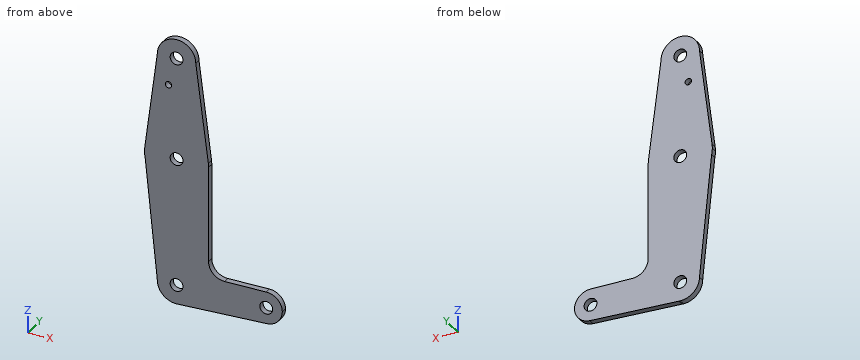
```python
from build123d import *

# Parameters (mm, degrees)
F0_R     = 3.175
F0_R_2   = 1.5875
F1_DEPTH = 3.048


with BuildPart() as f1:
    # F0 (on Front) → F1 (new body)
    with BuildSketch(Plane.XZ):
        with BuildLine():
            ThreePointArc((15.747457, 2.008289), (0, 15.875), (-15.747457, 2.008289))
            ThreePointArc((-15.747457, 2.008289), (-15.843082, 1.006168), (-15.875, 0))
            Line((-15.875, 0), (-15.560644, -3.143564))
            ThreePointArc((-15.560644, -3.143564), (1.579622, -15.796215), (15.875, 0))
            ThreePointArc((15.875, 0), (15.843082, 1.006168), (15.747457, 2.008289))
        make_face()
        Circle(F0_R, mode=Mode.SUBTRACT)
        with BuildLine():
            Line((-9.525, 50.8), (-15.747457, 2.008289))
            ThreePointArc((-15.747457, 2.008289), (0, 15.875), (15.747457, 2.008289))
            Line((15.747457, 2.008289), (9.525, 50.8))
            ThreePointArc((9.525, 50.8), (0, 41.275), (-9.525, 50.8))
        make_face()
        with Locations((-3.993369, 36.5252)):
            Circle(F0_R_2, mode=Mode.SUBTRACT)
        with BuildLine():
            Line((-15.560644, -3.143564), (-15.875, 0))
            ThreePointArc((-15.875, 0), (-15.796215, -1.579622), (-15.560644, -3.143564))
        make_face()
        with BuildLine():
            ThreePointArc((9.525, 50.8), (0, 60.325), (-9.525, 50.8))
            ThreePointArc((-9.525, 50.8), (0, 41.275), (9.525, 50.8))
        make_face()
        with Locations((0, 50.8)):
            Circle(F0_R, mode=Mode.SUBTRACT)
        with BuildLine():
            ThreePointArc((15.875, 0), (1.579622, -15.796215), (-15.560644, -3.143564))
            Line((-15.560644, -3.143564), (-9.525, -63.5))
            ThreePointArc((-9.525, -63.5), (0, -53.975), (9.525, -63.5))
            ThreePointArc((9.525, -63.5), (6.970557, -69.991299), (0.677344, -73.000886))
            Line((0.677344, -73.000886), (44.732405, -71.432475))
            ThreePointArc((44.732405, -71.432475), (36.513756, -63.641225), (44.45, -55.5625))
            Line((44.45, -55.5625), (23.8252, -55.5625))
            ThreePointArc((23.8252, -55.5625), (18.20356, -53.23394), (15.875, -47.6123))
            Line((15.875, -47.6123), (15.875, 0))
        make_face()
        with BuildLine():
            ThreePointArc((9.525, -63.5), (0, -53.975), (-9.525, -63.5))
            ThreePointArc((-9.525, -63.5), (-6.735192, -70.235192), (0, -73.025))
            Line((0, -73.025), (0.677344, -73.000886))
            ThreePointArc((0.677344, -73.000886), (6.970557, -69.991299), (9.525, -63.5))
        make_face()
        with Locations((0, -63.5)):
            Circle(F0_R, mode=Mode.SUBTRACT)
        with BuildLine():
            Line((0.677344, -73.000886), (0, -73.025))
            ThreePointArc((0, -73.025), (0.338886, -73.01897), (0.677344, -73.000886))
        make_face()
        with BuildLine():
            ThreePointArc((52.3875, -63.5), (50.06266, -57.88734), (44.45, -55.5625))
            ThreePointArc((44.45, -55.5625), (36.513756, -63.641225), (44.732405, -71.432475))
            ThreePointArc((44.732405, -71.432475), (50.161633, -69.01191), (52.3875, -63.5))
        make_face()
        with Locations((44.45, -63.5)):
            Circle(F0_R, mode=Mode.SUBTRACT)
    extrude(amount=F1_DEPTH)


solid = f1.part
```
Part model, mm, in its own coordinate system. Round coordinates to 2 decimals unless told otherwise and drop trailing zeros. Loops run counter-clockwise (first coordinate to the right, second up) from the corner with the lowest first, then second, coordinate; pieces in that order, holes last.
Item 1: Drop flat-ended pins along their axis: P1, Ø1.5, axis at y = -2.5, z = 7, coming from the +X side; P2, Ø1.5, axis at y = -1, z = -13, coming from the +X side (3 decimals); P3, Ø1.9, axis at x = -3.99, z = 36.53, coming from the -Y side; P4, Ø1.5, axis at x = 15, y = -2, coming from the -Z side. Give the stop position or say it passes through.
Item 2: Cut at A-A, the plane y = -0.5. State how many separate pieces and enclosed holes the cut face has, then the cut area to 3 significant figures.
Item 3: Drill centre lines: line 1 (Z direction, x = 44.45, y = -0.8) (1 decimal); line 2 (X direction, y = -0.85, z = -35) (3 decimals); line 3 (X direction, y = -2.3, z = 41). Where is each one in solid material? Low to high.
Item 4: Cut at C-C, the plane z = -18.5. Give the cut face in (x, y) (3 decimals), then the cut area to 3 significant figures.
Item 5: Cut at B-B, the plane x = -8. Give the cut face in (y, z), then the cut area to 3 significant figures.
A:
1. P1: stops at x = 15.21
1. P2: stops at x = 15.875
1. P3: passes through
1. P4: stops at z = -72.52
2. separate pieces: 1
2. enclosed holes: 5
2. area: 3,920 mm2
3. line 1: z = -71.4 to -66.7, -60.3 to -55.6
3. line 2: x = -12.375 to 15.875
3. line 3: x = -10.77 to 10.77
4. outline: (-14.025, -3.048) - (15.875, -3.048) - (15.875, 0) - (-14.025, 0) - close
4. area: 91.1 mm2
5. outline: (-3.05, -68.67) - (0, -68.67) - (0, 55.97) - (-3.05, 55.97) - close
5. area: 380 mm2
